```python
from build123d import *

# Parameters (mm, degrees)
SKETCH1_W                 = 101.6
SKETCH1_H                 = 34.036
BOSS_EXTRUDE1_DEPTH       = 2.54
CUT_EXTRUDE2_DEPTH        = 2.54
LPATTERN1_COUNT           = 2
LPATTERN1_PITCH           = 55
TAP_DRILL_FOR_6_32_TAP1_D = 2.7051
SKETCH2_R                 = 9.5
CUT_EXTRUDE3_DEPTH        = 2.54
SKETCH11_R                = 1.905
CUT_EXTRUDE5_DEPTH        = 2.54


with BuildPart() as part:
    # Sketch1 → Boss-Extrude1 (new body)
    with BuildSketch(Plane(origin=(0, 0, 0), x_dir=(1, 0, 0), z_dir=(0, 1, 0))):
        with Locations((50.8, 17.018)):
            Rectangle(SKETCH1_W, SKETCH1_H)
    extrude(amount=BOSS_EXTRUDE1_DEPTH)

    # Sketch7 → Cut-Extrude2 (cut)
    with BuildSketch(Plane(origin=(0, 2.54, 0), x_dir=(1, 0, 0), z_dir=(0, 1, 0))):
        Polygon((38.220191954, 3.75), (38.220191954, 18.75), (38.220191954, 34.036), (8.22019201, 34.036), (8.22019201, 3.75), align=None)
    cut_extrude2 = extrude(amount=-CUT_EXTRUDE2_DEPTH, mode=Mode.SUBTRACT)

    # LPattern1: Cut-Extrude2 ×2
    with Locations(*[(i * LPATTERN1_PITCH, 0, 0) for i in range(1, LPATTERN1_COUNT)]):
        add(cut_extrude2, mode=Mode.SUBTRACT)

    # Tap Drill for #6-32 Tap1 (through all)
    with Locations(Plane(origin=(0, 2.54, 0), x_dir=(1, 0, 0), z_dir=(0, 1, 0))):
        with Locations((43.875, 5.800000084), (57.725, 5.8)):
            Hole(TAP_DRILL_FOR_6_32_TAP1_D / 2)

    # Sketch2 → Cut-Extrude3 (cut)
    with BuildSketch(Plane(origin=(0, 2.54, 0), x_dir=(1, 0, 0), z_dir=(0, 1, 0))):
        with Locations(Location((50.8, 17.018, 0), (0, 0, 270))):
            Circle(SKETCH2_R)
    extrude(amount=-CUT_EXTRUDE3_DEPTH, mode=Mode.SUBTRACT)

    # Sketch11 → Cut-Extrude5 (cut)
    with BuildSketch(Plane(origin=(0, 2.54, 0), x_dir=(1, 0, 0), z_dir=(0, 1, 0))):
        with Locations(Location((4.43, 7.045, 0), (0, 0, 270))):
            Circle(SKETCH11_R)
        with Locations(Location((97.17, 7.045, 0), (0, 0, 270))):
            Circle(SKETCH11_R)
    extrude(amount=-CUT_EXTRUDE5_DEPTH, mode=Mode.SUBTRACT)


solid = part.part
```
Design review of the part built by this model. Coordinates are the model's own, in mm. A direction names the side the tool comes from. Round coordinates to 2 decimals unless told otherwise and drop trailing zeros. Write each loop counter-clockwise with the first axis right and the second up, starting at its lowest first coordinate (ties: lowest second). Pieces come first, ordered by that corner, then holes. Notation, with made-up numbers: (45.5, 33) -> (98.5, 33) arc R24 cw to (98.5, 48) -> close; hole circle Ø9 at (34.5, 53.25). An arc over 180 degrees is marked (long way). Write item = value, one per line. Start each with the question number.
1) Clearance check with flat-ended pins moving along their axes: pin 1 (0.8 mm diameter, centred on x = 81, y = 1, fed in from -Z); pin 2 (3 mm diameter, centred on x = 4.43, z = -7.045, fed in from -Y). State where each tip first meets the part, or that it passes through.
2) Tool access review of faces 4 (the face through (101.6, 1, -17)), 5 (the face through (78, 1, -3.75)): name each direction out of +Z, -Z, +X, -X, +Y, -Y from which nothing blocks a thin tool from reaching the whole face with its end or side.
3) Take a section at C-C, the plane y = 1.9. State the section outline as (x, z) points (3 decimals), plus the area to 3 significant figures.
4) Take a section at B-B, the plane z = -17. State the section outline as (x, y) points.
5) Wall thickness on probe 1 along X at (y, z) = (1.9, -28); probe 2 along X at (y, z) = (0.7, -9.5); probe 3 along X at (y, z) = (2.05, -14): over which ranges is each line inside the solid? List them lowest first. Write a range as from..to.
6) Mouldability with a two-part tool opening along Z and no side actions: class faces 1 (the face through (6.32, 1.29, -7.29)), 2 (the face through (97, 1, -34.036)), 3 (the face through (93.22, 1, -19)) as +Z half, -Z half, draft (parallel to the pull), parting line (faces both ways), or undercut.
7) Take a section at A-A, the plane x = 50.8. State the section outline as (y, z) points, plus the area to 3 significant figures.
8) Take a section at D-D, the plane x = 97.17. State the section outline as (y, z) points, plus the area to 3 significant figures.
Results list:
q1.pin_1 = -3.75
q1.pin_2 = through
q2.face_4 = +Z, -Z, +X, +Y, -Y
q2.face_5 = -Z, +Y, -Y
q3.outline = (0, -34.036) -> (8.22, -34.036) -> (8.22, -3.75) -> (38.22, -3.75) -> (38.22, -34.036) -> (63.22, -34.036) -> (63.22, -3.75) -> (93.22, -3.75) -> (93.22, -34.036) -> (101.6, -34.036) -> (101.6, 0) -> (0, 0) -> close; hole circle Ø3.81 at (4.43, -7.045); hole circle Ø19 at (50.8, -17.018); hole circle Ø2.705 at (43.875, -5.8); hole circle Ø2.705 at (57.725, -5.8); hole circle Ø3.81 at (97.17, -7.045)
q3.area = 1,320 mm²
q4.outline = (0, 0) -> (8.22, 0) -> (8.22, 2.54) -> (0, 2.54) -> close; (38.22, 0) -> (41.3, 0) -> (41.3, 2.54) -> (38.22, 2.54) -> close; (60.3, 0) -> (63.22, 0) -> (63.22, 2.54) -> (60.3, 2.54) -> close; (93.22, 0) -> (101.6, 0) -> (101.6, 2.54) -> (93.22, 2.54) -> close
q5.probe_1 = 0..8.22, 38.22..63.22, 93.22..101.6
q5.probe_2 = 0..8.22, 38.22..44.99, 56.61..63.22, 93.22..101.6
q5.probe_3 = 0..8.22, 38.22..41.79, 59.81..63.22, 93.22..101.6
q6.face_1 = undercut
q6.face_2 = -Z half
q6.face_3 = draft
q7.outline = (0, -34.04) -> (2.54, -34.04) -> (2.54, -26.52) -> (0, -26.52) -> close; (0, -7.52) -> (2.54, -7.52) -> (2.54, 0) -> (0, 0) -> close
q7.area = 38.2 mm²
q8.outline = (0, -34.04) -> (2.54, -34.04) -> (2.54, -8.95) -> (0, -8.95) -> close; (0, -5.14) -> (2.54, -5.14) -> (2.54, 0) -> (0, 0) -> close
q8.area = 76.8 mm²
